```python
from build123d import *

# Parameters (mm, degrees)
SKETCH1_R           = 85
SKETCH1_R_2         = 2.132457031
SKETCH1_R_3         = 2.1
BOSS_EXTRUDE1_DEPTH = 2.4
SKETCH2_R           = 58
BOSS_EXTRUDE2_DEPTH = 18.4
BOSS_EXTRUDE2_TAPER = 15
SKETCH3_R           = 50.15
CUT_EXTRUDE1_DEPTH  = 10
SKETCH4_R           = 48.5
CUT_EXTRUDE2_DEPTH  = 8.4


with BuildPart() as part:
    # Sketch1 → Boss-Extrude1 (new body)
    with BuildSketch(Plane(origin=(0, 0, 0), x_dir=(1, 0, 0), z_dir=(0, 1, 0))):
        with Locations(Location((0, 0, 0), (0, 0, 270))):
            Circle(SKETCH1_R)
        with Locations(Location((-75, 0, 0), (0, 0, 270))):
            Circle(SKETCH1_R_2, mode=Mode.SUBTRACT)
        with Locations(Location((0, 75, 0), (0, 0, 270))):
            Circle(SKETCH1_R_2, mode=Mode.SUBTRACT)
        with Locations(Location((75, 0, 0), (0, 0, 270))):
            Circle(SKETCH1_R_2, mode=Mode.SUBTRACT)
        with Locations(Location((0, -75, 0), (0, 0, 270))):
            Circle(SKETCH1_R_2, mode=Mode.SUBTRACT)
        with Locations(Location((-14, 0, 0), (0, 0, 270))):
            Circle(SKETCH1_R_3, mode=Mode.SUBTRACT)
        with Locations(Location((0, 14, 0), (0, 0, 270))):
            Circle(SKETCH1_R_3, mode=Mode.SUBTRACT)
        with Locations(Location((14, 0, 0), (0, 0, 270))):
            Circle(SKETCH1_R_3, mode=Mode.SUBTRACT)
        with Locations(Location((0, -14, 0), (0, 0, 270))):
            Circle(SKETCH1_R_3, mode=Mode.SUBTRACT)
    extrude(amount=BOSS_EXTRUDE1_DEPTH)

    # Sketch2 → Boss-Extrude2 (add)
    with BuildSketch(Plane(origin=(0, 2.4, 0), x_dir=(1, 0, 0), z_dir=(0, 1, 0))):
        Circle(SKETCH2_R)
    extrude(amount=BOSS_EXTRUDE2_DEPTH, taper=BOSS_EXTRUDE2_TAPER)

    # Sketch3 → Cut-Extrude1 (cut)
    with BuildSketch(Plane(origin=(0, 20.8, 0), x_dir=(1, 0, 0), z_dir=(0, 1, 0))):
        with Locations(Location((0, 0, 0), (0, 0, 270))):
            Circle(SKETCH3_R)
    extrude(amount=-CUT_EXTRUDE1_DEPTH, mode=Mode.SUBTRACT)

    # Sketch4 → Cut-Extrude2 (cut)
    with BuildSketch(Plane(origin=(0, 10.8, 0), x_dir=(1, 0, 0), z_dir=(0, 1, 0))):
        with Locations(Location((0, 0, 0), (0, 0, 270))):
            Circle(SKETCH4_R)
    extrude(amount=-CUT_EXTRUDE2_DEPTH, mode=Mode.SUBTRACT)


solid = part.part
```
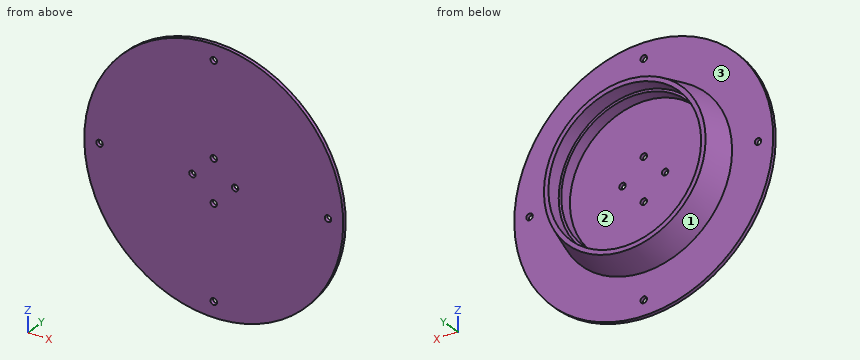
The model under review builds one solid part; all positions refer to its coordinate system, in mm. Face numbers are marked on the shaded views. Coordinates: 2 decimals unless noted, no trailing zeros. Write each loop counter-clockwise with the first axis right and the second up, starting at its lowest first coordinate (ties: lowest second). Pieces come first, ordered by that corner, then holes. Notation, with made-up numbers: (-18, -9.75) -> (8, -9.75) arc R9 cw to (8, -1.75) -> close; hole circle Ø6 at (53, 26). An arc over 180 degrees is marked (long way). One line per item, written item: value. Start each with the question number.
Q1. The part is to be moulded in two halves that separate along X. For the marked faces 1, 2 and 3, say which applies: +X half, -X half, draft (parallel to the pull), parting line (faces both ways), or undercut.
Q2. To check wall thickness, follow probe 1 along X at (y, z) = (1.9, 0); probe 2 along Y at (x, z) = (30, 34); probe 3 along X at (y, z) = (1, 75). State the ranges of each line that lie inside material, in increasing order.
Q3. Add section A-A, the plane x = 75. Give the boundary of the cut face in (y, z), then the cut area to 3 significant figures.
Q4. Add section C-C, the plane z = 0. Count the separate pieces of the cut face and the enclosed holes in it, then the cut area to 3 significant figures.
Q5. Add section B-B, the plane y = 18. Give the boundary of the cut face in (x, z).
Q6. Clearance check with flat-ended pins moving along their axes: P1, Ø5, axis at x = -26.5, y = 14, coming from the -Z side; P2, Ø12, axis at y = 3.5, z = 34.5, coming from the +X side; P3, Ø10, axis at x = 67, z = -22.5, coming from the +Y side. State where each tip first meets the part, or that it passes through.
Response:
1. face 1: parting line
1. face 2: undercut
1. face 3: draft
2. probe 1: -85 to -77.13, -72.87 to -16.1, -11.9 to 11.9, 16.1 to 72.87, 77.13 to 85
2. probe 2: 0 to 2.4
2. probe 3: -40 to -2.13, 2.13 to 40
3. outline: (0, -40) -> (2.4, -40) -> (2.4, -2.13) -> (0, -2.13) -> close; (0, 2.13) -> (2.4, 2.13) -> (2.4, 40) -> (0, 40) -> close
3. area: 182 mm²
4. separate pieces: 5
4. enclosed holes: 0
4. area: 593 mm²
5. outline: circle Ø107.64 at (0, 0); hole circle Ø100.3 at (0, 0)
6. P1: z = -49.58
6. P2: x = 80.04
6. P3: y = 2.4
